```python
from build123d import *

# Parameters (mm, degrees)
F0_R        = 15.875
F1_DEPTH    = 2.54
F2_W        = 0.2515364613
F2_H        = 31.190475449
F2_W_2      = 0.335381832
F2_H_2      = 30.6035578251
F2_W_3      = 0.4611494951
F2_H_3      = 29.9327941611
F2_H_4      = 28.8428049535
F2_W_4      = 0.5030720495
F2_H_5      = 27.5432020426
F2_W_5      = 0.5449950695
F2_H_6      = 25.9082177654
F2_W_6      = 0.7546087727
F2_H_7      = 24.1055423394
F2_H_8      = 19.7455827147
F3_DEPTH    = 1.27
F4_T1_DEPTH = 8.9452554821


# Not quite as in the source:
# - a fillet or chamfer that OpenCascade refuses, or shapes differently, is made with other operations: its cross-section is extruded or revolved along the edge and cut away or added


with BuildPart() as f1:
    # F0 (on Right) → F1 (new body)
    with BuildSketch(Plane.YZ):
        Circle(F0_R)
    extrude(amount=F1_DEPTH)

    # F2 (on Right) → F3 (join)
    with BuildSketch(Plane.YZ):
        with Locations((-0.5812076997, 0.0161286443)):
            Rectangle(F2_W, F2_H)
        with Locations((-1.7969654873, 0.1418972388)):
            Rectangle(F2_W_2, F2_H_2)
        with Locations((-3.4109887201, 0.0999742188)):
            Rectangle(F2_W_3, F2_H_3)
        with Locations((-4.9202053342, 0.0161286443)):
            Rectangle(F2_W_3, F2_H_4)
        with Locations((-6.366537651, -0.0048326328)):
            Rectangle(F2_W_4, F2_H_5)
        with Locations((-7.9805608839, -0.0257934444)):
            Rectangle(F2_W_5, F2_H_6)
        with Locations((-9.6784294583, 0.0790129416)):
            Rectangle(F2_W_6, F2_H_7)
        with Locations((-11.5439891815, 0.0370899215)):
            Rectangle(F2_W_5, F2_H_8)
        with Locations((0.5812076997, 0.0161286443)):
            Rectangle(F2_W, F2_H)
        with Locations((11.5439891815, 0.0370899215)):
            Rectangle(F2_W_5, F2_H_8)
        with Locations((1.7969654873, 0.1418972388)):
            Rectangle(F2_W_2, F2_H_2)
        with Locations((3.4109887201, 0.0999742188)):
            Rectangle(F2_W_3, F2_H_3)
        with Locations((4.9202053342, 0.0161286443)):
            Rectangle(F2_W_3, F2_H_4)
        with Locations((9.6784294583, 0.0790129416)):
            Rectangle(F2_W_6, F2_H_7)
        with Locations((7.9805608839, -0.0257934444)):
            Rectangle(F2_W_5, F2_H_6)
        with Locations((6.366537651, -0.0048326328)):
            Rectangle(F2_W_4, F2_H_5)
    extrude(amount=-F3_DEPTH)

    # F4: fillet of radius 5.08 on 1 edges, made by hand

    # F4_s2 → F4_t1 (cut)
    with BuildSketch(Plane.XZ.offset(-20.2167471289)):
        with BuildLine():
            ThreePointArc((0, 9.9098812789), (-0.9419048812, 8.345828338), (-1.27, 6.5497771138))
            Line((-1.27, 6.5497771138), (-1.27, 9.9098812789))
            Line((-1.27, 9.9098812789), (0, 9.9098812789))
        make_face()
    extrude(amount=F4_T1_DEPTH, mode=Mode.SUBTRACT)


solid = f1.part
```
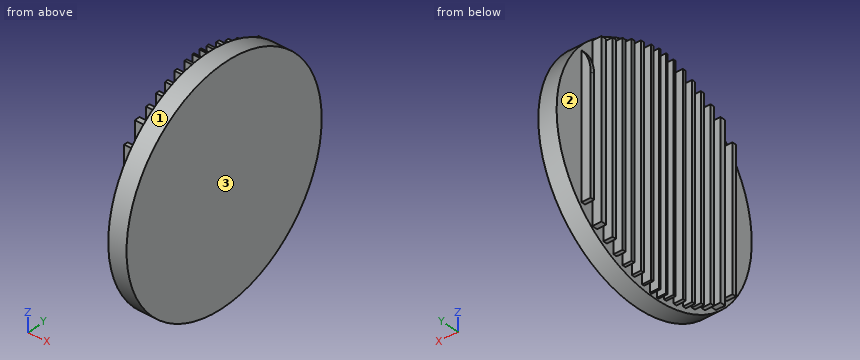
CAD build for the part. Positions are in the model's coordinates, mm. Face numbers are marked on the shaded views. Round coordinates to 2 decimals unless told otherwise and drop trailing zeros. Order: outer loops, then holes, each group sorted by start corner. A loop starts at its lowest first (then second) coordinate and runs counter-clockwise, first axis right, second up. Notation, with made-up numbers: (15.25, -1.75) -> (40.25, -1.75) arc R20 cw to (40.25, 21.25) -> close; hole circle Ø7 at (-21, 19.25). An arc over 180 degrees is marked (long way). One line per question, with ' | ' between items.
Q1. Drop flat-ended pins along their axis: pin 1 (6 mm diameter, centred on y = -4.5, z = 2, fed in from -X); pin 2 (1 mm diameter, centred on x = 1.5, y = 1.5, fed in from -Z); pin 3 (0.6 mm diameter, centred on x = -0.5, z = -3, fed in from +Y); pin 4 (0.6 mm diameter, centred on x = -1, z = -4, fed in from -Y). Give the stop position or say it passes through.
Completed:
pin 1: stops at x = -1.27 | pin 2: stops at z = -15.84 | pin 3: stops at y = 11.82 | pin 4: stops at y = -11.82
Q2. Slice it at B-B (y = 0). Write the cut outline in (x, z) (3 decimals), then the cut area to 3 significant figures.
Completed:
outline: (0, -15.875) -> (2.54, -15.875) -> (2.54, 15.875) -> (0, 15.875) -> close | area: 80.6 mm^2
Q3. Slice it at A-A (x = -0.4). Give the number of separate pieces and of enclosed holes in the cut face, then the cut area to 3 significant figures.
Completed:
separate pieces: 16 | enclosed holes: 0 | area: 204 mm^2
Q4. Slice it at C-C (x = 1.9). Write the cut outline in (y, z) (3 decimals).
Completed:
outline: circle Ø31.75 at (0, 0)
Q5. Probe probe 1 along Y at (x, z) = (0.8, -0.5); probe 2 along X at (y, z) = (8.5, 5); probe 3 along Z at (x, y) = (-0.8, -10). List the from-to ranges inside material, lowest first.
Completed:
probe 1: y = -15.87 to 15.87 | probe 2: x = 0 to 2.54 | probe 3: z = -11.97 to 12.13
Q6. Two-plate mould, pull along Y, no slides. Class the marked faces 1, 2 and 3: released by +Y, released by -Y, zero draft, split by the parting line, or undercut.
Completed:
face 1: split by the parting line | face 2: undercut | face 3: zero draft
